Model file for the job. Use its own axes, mm. Coordinates: 2 decimals unless noted, no trailing zeros. Write each loop counter-clockwise with the first axis right and the second up, starting at its lowest first coordinate (ties: lowest second). Pieces come first, ordered by that corner, then holes. Notation, with made-up numbers: (-5, 17) -> (49, 17) arc R29 ccw to (49, 48) -> close; hole circle Ø6 at (-36, 12). An arc over 180 degrees is marked (long way). Write item = value, one per line. Start each with the question number.
from build123d import *

# Parameters (mm, degrees)
SKETCH_1_W          = 140
SKETCH_1_H          = 220
SKETCH_1_R          = 1.75
EXTRUDE_1_DEPTH     = 3
SKETCH_2_R          = 1.75
SKETCH_2_R_2        = 20
CUT_EXTRUDE_1_DEPTH = 131.418556962
SKETCH_3_R          = 1.75
CUT_EXTRUDE_2_DEPTH = 131.418556962


with BuildPart() as part:
    # 草图1 → 凸台-拉伸1 (new body)
    with BuildSketch(Plane(origin=(0, 0, 0), x_dir=(1, 0, 0), z_dir=(0, 1, 0))):
        Rectangle(SKETCH_1_W, SKETCH_1_H)
        with Locations(Location((21.4, -74, 0), (0, 0, 270))):
            Circle(SKETCH_1_R, mode=Mode.SUBTRACT)
        with Locations(Location((21.4, -101.5, 0), (0, 0, 270))):
            Circle(SKETCH_1_R, mode=Mode.SUBTRACT)
        with Locations(Location((3.6, -101.5, 0), (0, 0, 270))):
            Circle(SKETCH_1_R, mode=Mode.SUBTRACT)
        with Locations(Location((3.6, -74, 0), (0, 0, 270))):
            Circle(SKETCH_1_R, mode=Mode.SUBTRACT)
    extrude(amount=EXTRUDE_1_DEPTH)

    # 草图2 → 切除-拉伸1 (cut, through all)
    with BuildSketch(Plane(origin=(0, 3, 0), x_dir=(1, 0, 0), z_dir=(0, 1, 0))):
        with Locations(Location((-35, 70, 0), (0, 0, 270))):
            Circle(SKETCH_2_R)
        with Locations(Location((35, 70, 0), (0, 0, 270))):
            Circle(SKETCH_2_R)
        with Locations(Location((-35, -70, 0), (0, 0, 270))):
            Circle(SKETCH_2_R)
        with Locations(Location((35, -70, 0), (0, 0, 270))):
            Circle(SKETCH_2_R)
        with Locations(Location((0, -30, 0), (0, 0, 270))):
            Circle(SKETCH_2_R_2)
    extrude(amount=-CUT_EXTRUDE_1_DEPTH, mode=Mode.SUBTRACT)

    # 草图3 → 切除-拉伸2 (cut, through all)
    with BuildSketch(Plane(origin=(0, 3, 0), x_dir=(1, 0, 0), z_dir=(0, 1, 0))):
        with Locations(Location((-39.3, 56, 0), (0, 0, 270))):
            Circle(SKETCH_3_R)
        with Locations(Location((-39.3, 4, 0), (0, 0, 270))):
            Circle(SKETCH_3_R)
        with Locations(Location((39.3, 4, 0), (0, 0, 270))):
            Circle(SKETCH_3_R)
        with Locations(Location((39.3, 56, 0), (0, 0, 270))):
            Circle(SKETCH_3_R)
        with Locations(Location((-56.213203436, 66.213203436, 0), (0, 0, 270))):
            Circle(SKETCH_3_R)
        with Locations(Location((56.213203436, 66.213203436, 0), (0, 0, 90))):
            Circle(SKETCH_3_R)
        with BuildLine():
            Line((-35, 80), (35, 80))
            ThreePointArc((35, 80), (59.748737342, 69.748737342), (70, 45))
            Line((70, 45), (70, 110))
            Line((70, 110), (-70, 110))
            Line((-70, 110), (-70, 45))
            ThreePointArc((-70, 45), (-59.748737342, 69.748737342), (-35, 80))
        make_face()
    extrude(amount=-CUT_EXTRUDE_2_DEPTH, mode=Mode.SUBTRACT)


solid = part.part
(1) Drill centre lines: line 1 along X through (y, z) = (1.15, 101.5); line 2 along X through (y, z) = (2, -70); line 3 along Z through (x, y) = (0.5, 2.85). Where is each one in solid material? Low to high.
(2) Saw through at B-B (x = 17.5). Give the cut face in (y, z), then the cut area to 3 significant figures.
(3) Drop flat-ended pins along their axis: pin 1 Ø1.5 at (x, y) = (-48, 1.5) entering from -Z; pin 2 Ø4 at (x, z) = (-56.21, -66.21) entering from +Y. Give the stop position or say it passes through.
(4) Saw through at A-A (z = 22). Give the cut face in (x, y).
(5) Mould opens along Z. For faces 1 (the face through (6.007, 1.521, 49.076)), 2 (the face through (59.475, 1.521, -70.019)), 3 (the face through (15, 3, 14)) say: released by +Z, released by -Z, zero draft, split by the parting line, or undercut.
(6) Saw through at D-D (x = -49.5). Give the cut face in (y, z), then the cut area to 3 significant figures.
(7) Saw through at C-C (y = 2.2). State how many separate pieces and enclosed holes the cut face has, then the cut area to 3 significant figures.
Returned:
q1.line_1 = -70 to 1.85, 5.35 to 19.65, 23.15 to 70
q1.line_2 = -59.49 to -36.75, -33.25 to 33.25, 36.75 to 59.49
q1.line_3 = -80 to 10.01, 49.99 to 110
q2.outline = (0, -80) -> (3, -80) -> (3, 20.32) -> (0, 20.32) -> close; (0, 39.68) -> (3, 39.68) -> (3, 110) -> (0, 110) -> close
q2.area = 512 mm2
q3.pin_1 = -77.79
q3.pin_2 = 3
q4.outline = (-70, 0) -> (-18.33, 0) -> (-18.33, 3) -> (-70, 3) -> close; (18.33, 0) -> (70, 0) -> (70, 3) -> (18.33, 3) -> close
q5.face_1 = undercut
q5.face_2 = released by -Z
q5.face_3 = zero draft
q6.outline = (0, -76.86) -> (3, -76.86) -> (3, 110) -> (0, 110) -> close
q6.area = 561 mm2
q7.separate_pieces = 1
q7.enclosed_holes = 15
q7.area = 24,700 mm2
